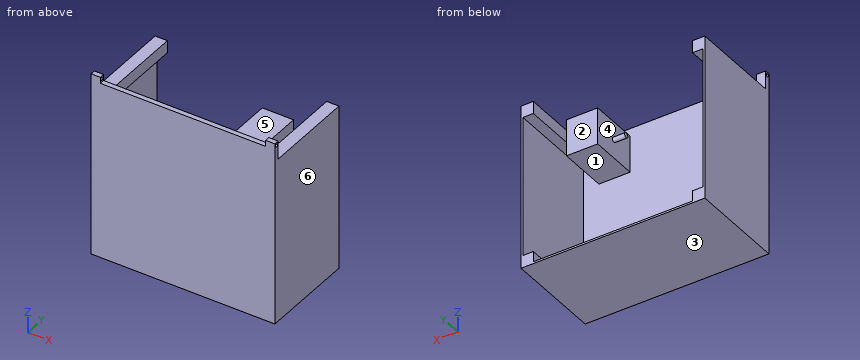
```python
from build123d import *

# Parameters (mm, degrees)
BOSS_EXTRUDE1_DEPTH     = 8
CUT_EXTRUDE1_DEPTH      = 213.282830205
CUT_EXTRUDE1_DEPTH_BACK = 213.282830205
SKETCH2_R               = 2.5
SKETCH3_W               = 20
SKETCH3_H               = 20
BOSS_EXTRUDE2_DEPTH     = 150
BOSS_EXTRUDE3_DEPTH     = 150
SKETCH5_W               = 51
SKETCH5_H               = 60
BOSS_EXTRUDE4_DEPTH     = 80
SKETCH7_R               = 4
BOSS_EXTRUDE5_DEPTH     = 20


with BuildPart() as part:
    # Sketch1 → Boss-Extrude1 (new body)
    with BuildSketch(Plane(origin=(0, 0, 0), x_dir=(1, 0, 0), z_dir=(0, 1, 0))):
        Polygon((135, -150), (150, -150), (150, 150), (-150, 150), (-150, -150), (-135, -150), (-135, -140), (135, -140), align=None)
    extrude(amount=BOSS_EXTRUDE1_DEPTH)

    # Sketch2 → Cut-Extrude1 (cut, two sides: drawn at the far end of the back side and taken through both)
    with BuildSketch(Plane(origin=(0, 0, 0), x_dir=(0, 0, -1), z_dir=(1, 0, 0)).offset(-CUT_EXTRUDE1_DEPTH_BACK)):
        with Locations((-145.033528283, 4)):
            Circle(SKETCH2_R)
    extrude(amount=CUT_EXTRUDE1_DEPTH + CUT_EXTRUDE1_DEPTH_BACK, mode=Mode.SUBTRACT)

    # Sketch3 → Boss-Extrude2 (add)
    with BuildSketch(Plane(origin=(0, 8, 0), x_dir=(1, 0, 0), z_dir=(0, 1, 0))):
        with Locations((-140, 140)):
            Rectangle(SKETCH3_W, SKETCH3_H)
        with Locations((140, 140)):
            Rectangle(SKETCH3_W, SKETCH3_H)
        with Locations((140, -110)):
            Rectangle(SKETCH3_W, SKETCH3_H)
        with Locations((-140, -110)):
            Rectangle(SKETCH3_W, SKETCH3_H)
    extrude(amount=BOSS_EXTRUDE2_DEPTH)

    # Sketch4 → Boss-Extrude3 (add)
    with BuildSketch(Plane(origin=(0, 8, 0), x_dir=(1, 0, 0), z_dir=(0, 1, 0))):
        Polygon((-147, 147), (-147, -117), (-150, -120), (-150, 150), (150, 150), (150, -120), (147, -117), (147, 147), align=None)
    extrude(amount=BOSS_EXTRUDE3_DEPTH)

    # Sketch5 → Boss-Extrude4 (add)
    with BuildSketch(Plane(origin=(0, 8, 0), x_dir=(1, 0, 0), z_dir=(0, 1, 0))):
        with Locations((96.729689643, -97.534797701)):
            Rectangle(SKETCH5_W, SKETCH5_H)
    extrude(amount=BOSS_EXTRUDE4_DEPTH)

    # Sketch7 → Boss-Extrude5 (add)
    with BuildSketch(Plane.ZY.offset(-71.229689643)):
        with Locations(Location((97.642468488, 48, 0), (0, 0, 180))):
            Circle(SKETCH7_R)
    extrude(amount=BOSS_EXTRUDE5_DEPTH)


solid = part.part
```
Model file for the job. Use its own axes, mm. Face numbers are marked on the shaded views. A direction names the side the tool comes from. Coordinates: 2 decimals unless noted, no trailing zeros. Loops run counter-clockwise (first coordinate to the right, second up) from the corner with the lowest first, then second, coordinate; pieces in that order, holes last. Notation, with made-up numbers: (79, -2) -> (136, -2) arc R13 cw to (136, 2) -> close; hole circle Ø4 at (-23, -8). An arc over 180 degrees is marked (long way). Answer as a JSON object with one key per item and string values.
Q1. Cut at C-C (x = 111). List the corners of the cut face in (y, z).
Report:
{"outline": "(0, -150) -> (158, -150) -> (158, -147) -> (8, -147) -> (8, 67.53) -> (88, 67.53) -> (88, 127.53) -> (8, 127.53) -> (8, 140) -> (0, 140) -> close"}
Q2. Flat gauge pins, fed straight in: P1, Ø1, axis at x = 52.5, y = 118, coming from the +Z side; P2, Ø5, axis at x = 102.5, z = 87, coming from the +Y side; P3, Ø4, axis at x = -20.5, z = -115, coming from the +Y side. Where does each tip first touch, or does it go through?
Report:
{"P1": "stops at z = -147", "P2": "stops at y = 88", "P3": "stops at y = 8"}
Q3. Pull direction X, two halves, no side cores. Call the marked faces 4, 5 and 6: released by +X, released by -X, zero draft, split by the parting line, or undercut.
Report:
{"face 4": "undercut", "face 5": "zero draft", "face 6": "released by +X"}
Q4. Cut at A-A (y = 48). List the corners of the cut face in (x, z), and give its area (3 significant figures).
Report:
{"outline": "(-150, -150) -> (150, -150) -> (150, 120) -> (130, 120) -> (130, 100) -> (147, 100) -> (147, -130) -> (130, -130) -> (130, -147) -> (-130, -147) -> (-130, -130) -> (-147, -130) -> (-147, 100) -> (-130, 100) -> (-130, 120) -> (-150, 120) -> close; (51.23, 93.64) -> (71.23, 93.64) -> (71.23, 67.53) -> (122.23, 67.53) -> (122.23, 127.53) -> (71.23, 127.53) -> (71.23, 101.64) -> (51.23, 101.64) -> close", "area": "6,980 mm2"}
Q5. 3-axis set-ups, long thin cutter, end or side, ignore diameter. For the marked faces 1, 2 and 3: which of +Z, -Z, +X, -X, +Y, -Y reach the whole face in a straight line?
Report:
{"face 1": "+Y", "face 2": "+Z, +Y", "face 3": "-Z, +X, -X, +Y, -Y"}
Q6. Cut at D-D (y = 64). List the corners of the cut face in (x, z).
Report:
{"outline": "(-150, -150) -> (150, -150) -> (150, 120) -> (130, 120) -> (130, 100) -> (147, 100) -> (147, -130) -> (130, -130) -> (130, -147) -> (-130, -147) -> (-130, -130) -> (-147, -130) -> (-147, 100) -> (-130, 100) -> (-130, 120) -> (-150, 120) -> close; (71.23, 67.53) -> (122.23, 67.53) -> (122.23, 127.53) -> (71.23, 127.53) -> close"}
Q7. Probe probe 1 along X at (y, z) = (25, 80); probe 2 along Z at (x, y) = (-140.5, 4); probe 3 along X at (y, z) = (65, -56.5). List the from-to ranges inside material, lowest first.
Report:
{"probe 1": "x = -150 to -147, 71.23 to 122.23, 147 to 150", "probe 2": "z = -150 to 142.53, 147.53 to 150", "probe 3": "x = -150 to -147, 147 to 150"}
Q8. Cut at B-B (z = -15). List the corners of the cut face in (x, y).
Report:
{"outline": "(-150, 0) -> (150, 0) -> (150, 158) -> (147, 158) -> (147, 8) -> (-147, 8) -> (-147, 158) -> (-150, 158) -> close"}
